Check sheet for the modelled part. Datum: model origin and axes. Units: mm. A direction names the side the tool comes from. Give positions to 0.01 mm unless a question says otherwise; leave off trailing zeros. Order: outer loops, then holes, each group sorted by start corner. A loop starts at its lowest first (then second) coordinate and runs counter-clockwise, first axis right, second up. Notation, with made-up numbers: M 70.25,38.25 L 111.25,38.25 A5 cw 111.25,43.25 Z; hole C 6.25,52.5 d6. An arc over 180 degrees is marked long. One line per question, with ' | ' between items. Start each with the question number.
```python
from build123d import *

# Parameters (mm, degrees)
EXTRUDE_1_DEPTH = 12.5
SKETCH_2_R      = 10
EXTRUDE_2_DEPTH = 80
CHAMFER_1_SIZE  = 2
CHAMFER_1_SIZE2 = 1.154700538


with BuildPart() as part:
    # Эскиз1 → Бобышка-Вытянуть1 (new body)
    with BuildSketch(Plane(origin=(0, 0, 0), x_dir=(1, 0, 0), z_dir=(0, 1, 0))):
        Polygon((14.801582536, -8.995173953), (15.190840422, 8.320959516), (0.389257887, 17.316133468), (-14.801582536, 8.995173953), (-15.190840422, -8.320959516), (-0.389257887, -17.316133468), align=None)
    extrude(amount=EXTRUDE_1_DEPTH)

    # Эскиз2 → Бобышка-Вытянуть2 (add)
    with BuildSketch(Plane(origin=(0, 12.5, 0), x_dir=(1, 0, 0), z_dir=(0, 1, 0))):
        Circle(SKETCH_2_R)
    extrude(amount=EXTRUDE_2_DEPTH)

    # Фаска1
    chamfer_1_edges = [part.edges().sort_by_distance(p)[0] for p in [
        (-7.790049154, 0, 12.818546492),
        (-14.996211479, 0, -0.337107218),
        (-7.206162325, 0, -13.155653711),
        (7.790049154, 0, -12.818546492),
        (14.996211479, 0, 0.337107218),
        (7.206162325, 0, 13.155653711),
    ]]
    chamfer_1_side = [part.faces().sort_by_distance(p)[0] for p in [
        (0, 0, 0),
    ]]
    chamfer(chamfer_1_edges, length=CHAMFER_1_SIZE, length2=CHAMFER_1_SIZE2, reference=chamfer_1_side[0])


solid = part.part
```
Item 1: Scan lines: probe 1 along Y at (x, z) = (11, -6.5); probe 2 along Y at (x, z) = (10, 10); probe 3 along X at (y, z) = (7, 9). Record each from-to range of solid material in increasing order. Write a range as [from, to].
Item 2: Set-up check for faces 1 (the face through (-6.626, 0.585, -12.349)), 2 (the face through (-2.17, 51.94, 9.76)): record each of +Z, -Z, +X, -X, +Y, -Y from which the full face is reachable in a straight line by a thin tool's end or side.
Item 3: Section check C-C, the plane z = 12. Record the cut outline in (x, y).
Item 4: Section check A-A, the plane x = 11.5. Record the cut outline in (y, z).
Item 5: Section check B-B, the plane y = 52. Record the cut outline in (x, z), then the cut area to 3 significant figures.
Item 6: Section check D-D, the plane z = 1. Record the cut outline in (x, y).
Item 7: Go/stop test with flat-tipped pins: P1, Ø10, axis at x = -1.5, y = 83, coming from the -Z side; P2, Ø8, axis at x = -4.5, y = 20.5, coming from the +Z side; P3, Ø10, axis at y = 26.5, z = 13.5, coming from the +X side. Record where each tip stops, or that it passes through.
Reported:
1) probe 1: y = [0, 12.5] | probe 2: y = [0.33, 12.5] | probe 3: x = [-14.07, 14.79]
2) face 1: -Z, -X, -Y | face 2: +Y
3) outline: M -9.14,1.15 L -5.29,0 L 5.15,0 L 9.32,1.15 L 9.32,12.5 L -9.14,12.5 Z
4) outline: M 0,-8.22 L 1.15,-10.56 L 12.5,-10.56 L 12.5,10.8 L 1.15,10.8 L 0,8.52 Z
5) outline: C 0,0 d20 | area: 314 mm^2
6) outline: M -15.03,1.15 L -13.03,0 L 12.98,0 L 14.98,1.15 L 14.98,12.5 L 9.95,12.5 L 9.95,92.5 L -9.95,92.5 L -9.95,12.5 L -15.03,12.5 Z
7) P1: stops at z = -10 | P2: stops at z = 9.99 | P3: stops at x = 5.27
